Input: part model. Units: mm. Frame: model coordinates. Face numbers are marked on the shaded views. A direction names the side the tool comes from. Give positions to 0.01 mm unless a question says otherwise; leave off trailing zeros. Loops run counter-clockwise (first coordinate to the right, second up) from the corner with the lowest first, then second, coordinate; pieces in that order, holes last. Notation, with made-up numbers: (-0.5, -11) -> (52.5, -11) arc R20 cw to (52.5, -1) -> close; hole circle Ø10 at (-6.5, -34.5). An arc over 180 degrees is marked (long way). Answer in a Markdown table with one row per item. Add a question column.
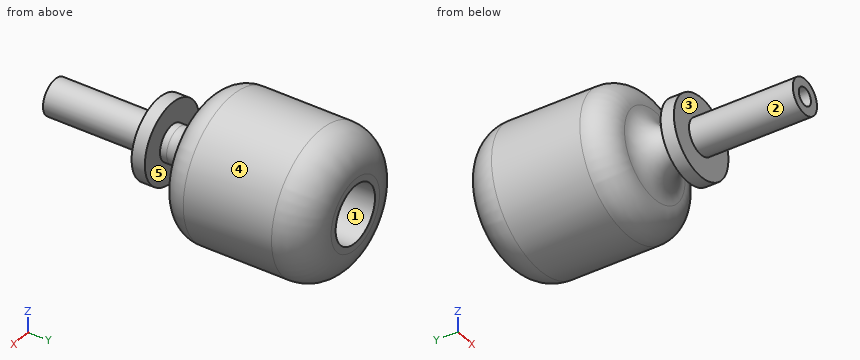
```python
from build123d import *

# Parameters (mm, degrees)
SKETCH_2_R          = 6.5
CUT_EXTRUDE_1_DEPTH = 30
CUT_EXTRUDE_2_REACH = 73.666
SKETCH_3_R          = 2
EXTRUDE_START       = -23.5
SKETCH_4_R          = 9
SKETCH_4_R_2        = 2
EXTRUDE_4_DEPTH     = 3


with BuildPart() as part:
    # 스케치1 → 회전2 (revolve)
    with BuildSketch(Plane.XY, mode=Mode.PRIVATE) as revolve_2_sk:
        with BuildLine():
            Line((0, 54.747282219), (-8, 54.747282219))
            ThreePointArc((-8, 54.747282219), (-13.656854249, 52.404136469), (-16, 46.747282219))
            Line((-16, 46.747282219), (-16, 26.747282219))
            ThreePointArc((-16, 26.747282219), (-14.242640687, 22.504641532), (-10, 20.747282219))
            ThreePointArc((-10, 20.747282219), (-5.757359313, 18.989922906), (-4, 14.747282219))
            Line((-4, 14.747282219), (-4, -13.252717781))
            Line((-4, -13.252717781), (0, -13.252717781))
            Line((0, -13.252717781), (0, 54.747282219))
        make_face()
    revolve(revolve_2_sk.sketch.rotate(Axis((0, 0, 0), (0, 1, 0)), 270), axis=Axis((0, 0, 0), (0, 1, 0)))

    # 스케치2 → 컷-돌출1 (cut)
    with BuildSketch(Plane(origin=(0, 54.747282219, 0), x_dir=(1, 0, 0), z_dir=(0, 1, 0))):
        with Locations(Location((0, 0, 0), (0, 0, 270))):
            Circle(SKETCH_2_R)
    extrude(amount=-CUT_EXTRUDE_1_DEPTH, mode=Mode.SUBTRACT)

    # 스케치3 → 컷-돌출2 (cut, up to next)
    with BuildSketch(Plane.XZ.offset(13.252717781), mode=Mode.PRIVATE) as cut_extrude_2_sk1:
        with Locations(Location((0, 0, 0), (0, 0, 270))):
            Circle(SKETCH_3_R)
    cut_extrude_2_tool1 = extrude(cut_extrude_2_sk1.sketch, amount=-CUT_EXTRUDE_2_REACH, mode=Mode.PRIVATE) & part.part
    add(cut_extrude_2_tool1.solids().sort_by_distance((0, -13.252718, 0))[0], mode=Mode.SUBTRACT)

    # 스케치4 → 보스-돌출4 (add)
    with BuildSketch(Plane.XZ.offset(13.252717781).offset(EXTRUDE_START)):
        with Locations(Location((0, 0, 0), (0, 0, 270))):
            Circle(SKETCH_4_R)
        with Locations(Location((0, 0, 0), (0, 0, 270))):
            Circle(SKETCH_4_R_2, mode=Mode.SUBTRACT)
    extrude(amount=-EXTRUDE_4_DEPTH)


solid = part.part
```
1) Pull-direction query (Y, two-part tool) for the marked faces 3, 4 and 5; classes: +Y half, -Y half, draft (parallel to the pull), parting line (faces both ways), or undercut.
2) Pin query (flat end, axial travel): pin 1 (3 mm diameter, centred on x = -1, y = 13, fed in from -Z); pin 2 (4 mm diameter, centred on y = 13, z = 8, fed in from +X); pin 3 (17 mm diameter, centred on x = 0, z = 0, fed in from +Y); pin 4 (1.5 mm diameter, centred on y = 14, z = 10.5, fed in from +X). Return the tip coordinate at first contact, or that it passes through.
3) Reachability of the marked faces 1 and 2 from +Z, -Z, +X, -X, +Y, -Y: full face, straight path, thin tool, end or side. Return the list, or none.
4) Section B-B on y = 3. Output: boundary loops of the cut face in (x, z), and give its area (3 significant figures).
5) Section A-A on y = 30.5. Output: boundary loops of the cut face in (x, z), and give its area (3 significant figures).
6) Material intervals for line 1 along X through (y, z) = (45.75, 0); line 2 along X through (y, z) = (4, 0); line 3 along Y through (x, z) = (6, 3.5), sorted ascending.
Working result:
| question | item | result |
|---|---|---|
| 1 | face 3 | -Y half |
| 1 | face 4 | draft |
| 1 | face 5 | undercut |
| 2 | pin 1 | stops at z = -9 |
| 2 | pin 2 | stops at x = 6.71 |
| 2 | pin 3 | stops at y = 54.75 |
| 2 | pin 4 | passes through |
| 3 | face 1 | +Y |
| 3 | face 2 | -Y |
| 4 | outline | circle Ø8 at (0, 0); hole circle Ø4 at (0, 0) |
| 4 | area | 37.7 mm2 |
| 5 | outline | circle Ø32 at (0, 0); hole circle Ø13 at (0, 0) |
| 5 | area | 672 mm2 |
| 6 | line 1 | x = -16 to -6.5, 6.5 to 16 |
| 6 | line 2 | x = -4 to -2, 2 to 4 |
| 6 | line 3 | y = 10.25 to 13.25, 19.91 to 54.75 |
